from build123d import *
from OCP.BRepFilletAPI import BRepFilletAPI_MakeChamfer

# Parameters (mm, degrees)
SKETCH1_W            = 45
SKETCH1_H            = 25
SKETCH1_R            = 5.1
SKETCH1_R_2          = 3.5
BOSS_EXTRUDE1_DEPTH  = 5
CUT_EXTRUDE3_DEPTH   = 5.5
MIRROR2_COPY_1_DEPTH = 5.5
CHAMFER1_SIZE        = 0.25
CHAMFER1_SIZE2       = 0.301404498


with BuildPart() as part:
    # Sketch1 → Boss-Extrude1 (new body)
    with BuildSketch(Plane(origin=(0, 0, 0), x_dir=(1, 0, 0), z_dir=(0, 1, 0))):
        Rectangle(SKETCH1_W, SKETCH1_H)
        with Locations(Location((-10, 0, 0), (0, 0, 270))):
            Circle(SKETCH1_R, mode=Mode.SUBTRACT)
        with Locations(Location((10, 0, 0), (0, 0, 270))):
            Circle(SKETCH1_R, mode=Mode.SUBTRACT)
        with Locations(Location((0, -4, 0), (0, 0, 270))):
            Circle(SKETCH1_R_2, mode=Mode.SUBTRACT)
    extrude(amount=BOSS_EXTRUDE1_DEPTH)

    # Sketch4 → Cut-Extrude3 (cut)
    with BuildSketch(Plane(origin=(-17.5, 0, -17.5), x_dir=(0, -1, 0), z_dir=(-0.7071067811865488, 0, -0.7071067811865464))):
        Polygon((-5, 8.671067812), (-5, 5.471067812), (-2.5, 5.871067812), (0, 5.471067812), (0, 8.671067812), (-2.5, 8.271067812), align=None)
    cut_extrude3 = extrude(amount=-CUT_EXTRUDE3_DEPTH, mode=Mode.SUBTRACT)

    # Mirror1: Cut-Extrude3 across plane
    add(cut_extrude3.mirror(Plane.XY), mode=Mode.SUBTRACT)

    # Mirror2: Cut-Extrude3 across plane
    add(cut_extrude3.mirror(Plane(origin=(0, 0, 0), x_dir=(0, 0, 1), z_dir=(1, 0, 0))), mode=Mode.SUBTRACT)

    # Mirror2 copy 1 sketch → Mirror2 copy 1 (cut)
    with BuildSketch(Plane(origin=(17.5, 0, 17.5), x_dir=(0, -1, 0), z_dir=(0.7071067811865488, 0, 0.7071067811865464))):
        Polygon((-5, 8.671067812), (-5, 5.471067812), (-2.5, 5.871067812), (0, 5.471067812), (0, 8.671067812), (-2.5, 8.271067812), align=None)
    extrude(amount=-MIRROR2_COPY_1_DEPTH, mode=Mode.SUBTRACT)

    # Chamfer1: one chamfer whose edges measure the first distance from different faces: ONE call of the kernel's chamfer builder (chamfer() names one face for all edges)
    chamfer1_edges_1 = [part.edges().sort_by_distance(p)[0] for p in [
        (22.5, 5, 0),
        (22.5, 0, 0),
        (18.610912703, 0, 8.610912703),
        (18.610912703, 5, 8.610912703),
        (-10, 0, -5.1),
        (-10, 5, -5.1),
        (10, 0, -5.1),
        (10, 5, -5.1),
        (0, 0, 0.5),
        (0, 5, 0.5),
        (-22.5, 0, 0),
        (-22.5, 5, 0),
        (-18.610912703, 0, -8.610912703),
        (-18.610912703, 5, -8.610912703),
        (0, 0, 12.5),
        (0, 5, 12.5),
        (-18.610912703, 5, 8.610912703),
        (-18.610912703, 0, 8.610912703),
        (0, 0, -12.5),
        (0, 5, -12.5),
        (18.610912703, 5, -8.610912703),
        (18.610912703, 0, -8.610912703),
    ]]
    chamfer1_edges_2 = [part.edges().sort_by_distance(p)[0] for p in [
        (21.121141777, 5, 8.858400077),
    ]]
    chamfer1_side_2 = [part.faces().sort_by_distance(p)[0] for p in [
        (21.049281331, 3.729674797, 9.073981413),
    ]]
    chamfer1_edges_3 = [part.edges().sort_by_distance(p)[0] for p in [
        (21.121141777, 0, 8.858400077),
        (-21.121141777, 0, -8.858400077),
        (-18.858400077, 0, 11.121141777),
        (18.858400077, 0, -11.121141777),
    ]]
    chamfer1_side_3 = [part.faces().sort_by_distance(p)[0] for p in [
        (0, 0, -0.178389984),
    ]]
    chamfer1_edges_4 = [part.edges().sort_by_distance(p)[0] for p in [
        (18.858400077, 0, 11.121141777),
    ]]
    chamfer1_side_4 = [part.faces().sort_by_distance(p)[0] for p in [
        (19.073981413, 1.270325203, 11.049281331),
    ]]
    chamfer1_edges_5 = [part.edges().sort_by_distance(p)[0] for p in [
        (18.858400077, 5, 11.121141777),
        (-18.858400077, 5, -11.121141777),
        (-21.121141777, 5, 8.858400077),
        (21.121141777, 5, -8.858400077),
    ]]
    chamfer1_side_5 = [part.faces().sort_by_distance(p)[0] for p in [
        (0, 5, -0.178389984),
    ]]
    chamfer1_edges_6 = [part.edges().sort_by_distance(p)[0] for p in [
        (-21.121141777, 5, -8.858400077),
    ]]
    chamfer1_side_6 = [part.faces().sort_by_distance(p)[0] for p in [
        (-21.049281331, 3.729674797, -9.073981413),
    ]]
    chamfer1_edges_7 = [part.edges().sort_by_distance(p)[0] for p in [
        (-18.858400077, 0, -11.121141777),
    ]]
    chamfer1_side_7 = [part.faces().sort_by_distance(p)[0] for p in [
        (-19.073981413, 1.270325203, -11.049281331),
    ]]
    chamfer1_edges_8 = [part.edges().sort_by_distance(p)[0] for p in [
        (-21.121141777, 0, 8.858400077),
    ]]
    chamfer1_side_8 = [part.faces().sort_by_distance(p)[0] for p in [
        (-21.049281331, 1.270325203, 9.073981413),
    ]]
    chamfer1_edges_9 = [part.edges().sort_by_distance(p)[0] for p in [
        (-18.858400077, 5, 11.121141777),
    ]]
    chamfer1_side_9 = [part.faces().sort_by_distance(p)[0] for p in [
        (-19.073981413, 3.729674797, 11.049281331),
    ]]
    chamfer1_edges_10 = [part.edges().sort_by_distance(p)[0] for p in [
        (21.121141777, 0, -8.858400077),
    ]]
    chamfer1_side_10 = [part.faces().sort_by_distance(p)[0] for p in [
        (21.049281331, 1.270325203, -9.073981413),
    ]]
    chamfer1_edges_11 = [part.edges().sort_by_distance(p)[0] for p in [
        (18.858400077, 5, -11.121141777),
    ]]
    chamfer1_side_11 = [part.faces().sort_by_distance(p)[0] for p in [
        (19.073981413, 3.729674797, -11.049281331),
    ]]
    chamfer1 = BRepFilletAPI_MakeChamfer(part.part.solid().wrapped)
    for e in chamfer1_edges_1:
        chamfer1.Add(CHAMFER1_SIZE, e.wrapped)
    for e in chamfer1_edges_2:
        chamfer1.Add(CHAMFER1_SIZE, CHAMFER1_SIZE2, e.wrapped, chamfer1_side_2[0].wrapped)  # the first distance lies on this face
    for e in chamfer1_edges_3:
        chamfer1.Add(CHAMFER1_SIZE, CHAMFER1_SIZE2, e.wrapped, chamfer1_side_3[0].wrapped)  # the first distance lies on this face
    for e in chamfer1_edges_4:
        chamfer1.Add(CHAMFER1_SIZE, CHAMFER1_SIZE2, e.wrapped, chamfer1_side_4[0].wrapped)  # the first distance lies on this face
    for e in chamfer1_edges_5:
        chamfer1.Add(CHAMFER1_SIZE, CHAMFER1_SIZE2, e.wrapped, chamfer1_side_5[0].wrapped)  # the first distance lies on this face
    for e in chamfer1_edges_6:
        chamfer1.Add(CHAMFER1_SIZE, CHAMFER1_SIZE2, e.wrapped, chamfer1_side_6[0].wrapped)  # the first distance lies on this face
    for e in chamfer1_edges_7:
        chamfer1.Add(CHAMFER1_SIZE, CHAMFER1_SIZE2, e.wrapped, chamfer1_side_7[0].wrapped)  # the first distance lies on this face
    for e in chamfer1_edges_8:
        chamfer1.Add(CHAMFER1_SIZE, CHAMFER1_SIZE2, e.wrapped, chamfer1_side_8[0].wrapped)  # the first distance lies on this face
    for e in chamfer1_edges_9:
        chamfer1.Add(CHAMFER1_SIZE, CHAMFER1_SIZE2, e.wrapped, chamfer1_side_9[0].wrapped)  # the first distance lies on this face
    for e in chamfer1_edges_10:
        chamfer1.Add(CHAMFER1_SIZE, CHAMFER1_SIZE2, e.wrapped, chamfer1_side_10[0].wrapped)  # the first distance lies on this face
    for e in chamfer1_edges_11:
        chamfer1.Add(CHAMFER1_SIZE, CHAMFER1_SIZE2, e.wrapped, chamfer1_side_11[0].wrapped)  # the first distance lies on this face
    add(Compound.cast(chamfer1.Shape()), mode=Mode.REPLACE)


solid = part.part
Design review of the part built by this model. Coordinates are the model's own, in mm. A direction names the side the tool comes from. Coordinates: 2 decimals unless noted, no trailing zeros. Loops run counter-clockwise (first coordinate to the right, second up) from the corner with the lowest first, then second, coordinate; pieces in that order, holes last.
Item 1: Add section B-B (y = 3.1). Write out the cut boundary in (x, z).
Completed:
outline: (-22.5, -10.67) - (-19.53, -7.69) - (-17.69, -9.53) - (-20.67, -12.5) - (20.67, -12.5) - (17.69, -9.53) - (19.53, -7.69) - (22.5, -10.67) - (22.5, 10.67) - (19.53, 7.69) - (17.69, 9.53) - (20.67, 12.5) - (-20.67, 12.5) - (-17.69, 9.53) - (-19.53, 7.69) - (-22.5, 10.67) - close; hole circle Ø10.2 at (-10, 0); hole circle Ø7 at (0, 4); hole circle Ø10.2 at (10, 0)
Item 2: Add section A-A (x = 0). Write out the cut boundary in (y, z).
Completed:
outline: (0, -12.25) - (0.25, -12.5) - (4.75, -12.5) - (5, -12.25) - (5, 0.25) - (4.75, 0.5) - (0.25, 0.5) - (0, 0.25) - close; (0, 7.75) - (0.25, 7.5) - (4.75, 7.5) - (5, 7.75) - (5, 12.25) - (4.75, 12.5) - (0.25, 12.5) - (0, 12.25) - close
Item 3: Wall thickness on L1, parallel to X at y = 1.65, z = 0; L2, parallel to Z at x = 18, y = 3.8; L3, parallel to X at y = 2.5, z = -3.5: over which ranges is each line inside the solid? List them lowest first.
Completed:
L1: x = -22.5 to -15.1, -4.9 to 4.9, 15.1 to 22.5
L2: z = -12.5 to -9.99, -9.22 to 9.22, 9.99 to 12.5
L3: x = -22.5 to -13.71, -6.29 to 6.29, 13.71 to 22.5
Item 4: Add section D-D (z = 3.25). Give the number of separate pieces and of enclosed holes in the cut face, and give its area (3 significant figures).
Completed:
separate pieces: 4
enclosed holes: 0
area: 112 mm2
Item 5: Clearance check with a flat-ended pin moving along its axis: pin 1 (13.5 mm diameter, centred on x = 10, z = 0, fed in from -Y). State where the tip first meets the part, or that it passes through.
Completed:
pin 1: stops at y = 0
Item 6: For faces 1 (the flat face through (19.18, 3.62, 11.13)), 2 (the flat face through (19.18, 1.39, 11.13)), 3 (the cylindrical face through (15, 2, -1)), list the 3-axis set-ups (+Z, -Z, +X, -X, +Y, -Y) from which the entire face can be reached by the end or side of a thin tool; tool diameter is ignored.
Completed:
face 1: +Y
face 2: -Y
face 3: +Y, -Y
Item 7: Draft analysis for pull direction X (two halves, no side actions). For faces 4 (the flat face through (-18.49, 0.13, -8.56)), 5 (the flat face through (22.5, 2, 0)), 6 (the flat face through (0, 2, 12.5)), state which applies: pulls with the +X half, pulls with the -X half, needs draft (parallel to the pull), parting line crosses it, or undercut.
Completed:
face 4: undercut
face 5: pulls with the +X half
face 6: needs draft
Item 8: Add section C-C (x = -10). Write out the cut boundary in (y, z).
Completed:
outline: (0, -12.25) - (0.25, -12.5) - (4.75, -12.5) - (5, -12.25) - (5, -5.35) - (4.75, -5.1) - (0.25, -5.1) - (0, -5.35) - close; (0, 5.35) - (0.25, 5.1) - (4.75, 5.1) - (5, 5.35) - (5, 12.25) - (4.75, 12.5) - (0.25, 12.5) - (0, 12.25) - close
